Check sheet for the modelled part. Datum: model origin and axes. Units: mm. A direction names the side the tool comes from. Coordinates: 2 decimals unless noted, no trailing zeros. Loops run counter-clockwise (first coordinate to the right, second up) from the corner with the lowest first, then second, coordinate; pieces in that order, holes last.
```python
from build123d import *

# Parameters (mm, degrees)
SKETCH1_R               = 10
BOSS_EXTRUDE1_DEPTH     = 61
SKETCH3_W               = 66
SKETCH3_H               = 1.5
SKETCH4_W               = 43
SKETCH4_H               = 1.5
SKETCH5_W               = 24
SKETCH5_H               = 2.5
SKETCH6_W               = 39.5
SKETCH6_H               = 1
SKETCH7_W               = 27
SKETCH7_H               = 1.5
SKETCH8_W               = 1.1
SKETCH8_H               = 0.6
SKETCH9_W               = 1.1
SKETCH9_H               = 0.65
SKETCH10_W              = 1.1
SKETCH10_H              = 0.65
CUT_EXTRUDE1_DEPTH      = 63.617888818
CUT_EXTRUDE1_DEPTH_BACK = 63.617888818
SKETCH11_W              = 12
SKETCH11_H              = 12
CUT_EXTRUDE2_DEPTH      = 2.5


with BuildPart() as part:
    # Sketch1 → Boss-Extrude1 (new, symmetric)
    with BuildSketch(Plane.XY):
        with Locations(Location((0, 0, 0), (0, 0, 180))):
            Circle(SKETCH1_R)
    extrude(amount=BOSS_EXTRUDE1_DEPTH, both=True)

    # Sketch3 → Cut-Revolve1 (revolve, cut)
    with BuildSketch(Plane(origin=(0, 0, 0), x_dir=(0, 0, -1), z_dir=(1, 0, 0)), mode=Mode.PRIVATE) as cut_revolve1_sk:
        with Locations((28, 9.25)):
            Rectangle(SKETCH3_W, SKETCH3_H)
    revolve(cut_revolve1_sk.sketch.rotate(Axis((0, 0, 0), (0, 0, -1)), 270), axis=Axis((0, 0, 0), (0, 0, -1)), mode=Mode.SUBTRACT)

    # Sketch4 → Cut-Revolve2 (revolve, cut)
    with BuildSketch(Plane(origin=(0, 0, 0), x_dir=(0, 0, -1), z_dir=(1, 0, 0)), mode=Mode.PRIVATE) as cut_revolve2_sk:
        with Locations((-39.5, 9.25)):
            Rectangle(SKETCH4_W, SKETCH4_H)
    revolve(cut_revolve2_sk.sketch.rotate(Axis((0, 0, 0), (0, 0, 1)), 90), axis=Axis((0, 0, 0), (0, 0, 1)), mode=Mode.SUBTRACT)

    # Sketch5 → Cut-Revolve3 (revolve, cut)
    with BuildSketch(Plane(origin=(0, 0, 0), x_dir=(0, 0, -1), z_dir=(1, 0, 0)), mode=Mode.PRIVATE) as cut_revolve3_sk:
        with Locations((-49, 7.25)):
            Rectangle(SKETCH5_W, SKETCH5_H)
    revolve(cut_revolve3_sk.sketch.rotate(Axis((0, 0, 0), (0, 0, 1)), 90), axis=Axis((0, 0, 0), (0, 0, 1)), mode=Mode.SUBTRACT)

    # Sketch6 → Cut-Revolve4 (revolve, cut)
    with BuildSketch(Plane(origin=(0, 0, 0), x_dir=(0, 0, -1), z_dir=(1, 0, 0)), mode=Mode.PRIVATE) as cut_revolve4_sk:
        with Locations((41.25, 8)):
            Rectangle(SKETCH6_W, SKETCH6_H)
    revolve(cut_revolve4_sk.sketch.rotate(Axis((0, 0, 0), (0, 0, -1)), 90), axis=Axis((0, 0, 0), (0, 0, -1)), mode=Mode.SUBTRACT)

    # Sketch7 → Cut-Revolve5 (revolve, cut)
    with BuildSketch(Plane(origin=(0, 0, 0), x_dir=(0, 0, -1), z_dir=(1, 0, 0)), mode=Mode.PRIVATE) as cut_revolve5_sk:
        with Locations((47.5, 6.75)):
            Rectangle(SKETCH7_W, SKETCH7_H)
    revolve(cut_revolve5_sk.sketch.rotate(Axis((0, 0, 0), (0, 0, -1)), 90), axis=Axis((0, 0, 0), (0, 0, -1)), mode=Mode.SUBTRACT)

    # Sketch8 → Cut-Revolve6 (revolve, cut)
    with BuildSketch(Plane(origin=(0, 0, 0), x_dir=(0, 0, -1), z_dir=(1, 0, 0)), mode=Mode.PRIVATE) as cut_revolve6_sk:
        with Locations((30.95, 7.2)):
            Rectangle(SKETCH8_W, SKETCH8_H)
    revolve(cut_revolve6_sk.sketch.rotate(Axis((0, 0, 0), (0, 0, -1)), 90), axis=Axis((0, 0, 0), (0, 0, -1)), mode=Mode.SUBTRACT)

    # Sketch9 → Cut-Revolve7 (revolve, cut)
    with BuildSketch(Plane(origin=(0, 0, 0), x_dir=(0, 0, -1), z_dir=(1, 0, 0)), mode=Mode.PRIVATE) as cut_revolve7_sk:
        with Locations((5.45, 8.175)):
            Rectangle(SKETCH9_W, SKETCH9_H)
    revolve(cut_revolve7_sk.sketch.rotate(Axis((0, 0, 0), (0, 0, -1)), 90), axis=Axis((0, 0, 0), (0, 0, -1)), mode=Mode.SUBTRACT)

    # Sketch10 → Cut-Revolve8 (revolve, cut)
    with BuildSketch(Plane(origin=(0, 0, 0), x_dir=(0, 0, -1), z_dir=(1, 0, 0)), mode=Mode.PRIVATE) as cut_revolve8_sk:
        with Locations((-34.45, 8.175)):
            Rectangle(SKETCH10_W, SKETCH10_H)
    revolve(cut_revolve8_sk.sketch.rotate(Axis((0, 0, 0), (0, 0, 1)), 90), axis=Axis((0, 0, 0), (0, 0, 1)), mode=Mode.SUBTRACT)

    # Sketch11 → Cut-Extrude1 (cut, two sides: drawn at the far end of the back side and taken through both)
    with BuildSketch(Plane(origin=(0, 0, 0), x_dir=(0, 0, -1), z_dir=(1, 0, 0)).offset(-CUT_EXTRUDE1_DEPTH_BACK)):
        with Locations((55, 0)):
            Rectangle(SKETCH11_W, SKETCH11_H)
    extrude(amount=CUT_EXTRUDE1_DEPTH + CUT_EXTRUDE1_DEPTH_BACK, mode=Mode.SUBTRACT)

    # Sketch12 → Cut-Extrude2 (cut)
    with BuildSketch(Plane(origin=(0, 8.5, 0), x_dir=(1, 0, 0), z_dir=(0, 1, 0))):
        with BuildLine():
            Line((2, -31.5), (2, -20.5))
            ThreePointArc((2, -20.5), (0, -18.5), (-2, -20.5))
            Line((-2, -20.5), (-2, -31.5))
            ThreePointArc((-2, -31.5), (0, -33.5), (2, -31.5))
        make_face()
    extrude(amount=-CUT_EXTRUDE2_DEPTH, mode=Mode.SUBTRACT)


solid = part.part
```
1) Set-up check for faces 1 (the flat face through (-7, 2, -31.5)), 2 (the flat face through (-4.5, 7.4, 18)), 3 (the cylindrical face through (5.723, -1.802, -41.605)): record each of +Z, -Z, +X, -X, +Y, -Y from which the full face is reachable in a straight line by a thin tool's end or side.
Answer sheet:
face 1: none
face 2: +Z
face 3: -Z
2) Section check B-B on z = 43. Enter the section's corners in (x, y).
Answer sheet:
outline: circle Ø12 at (0, 0)
3) Section check A-A on z = -2.5. Enter the section's corners in (x, y).
Answer sheet:
outline: circle Ø17 at (0, 0)
4) Scan lines: line 1 (Z direction, x = 2.25, y = -8); line 2 (Z direction, x = 9, y = 1); line 3 (X direction, y = 0.25, z = 44). Record each from-to range of solid material in increasing order.
Answer sheet:
line 1: z = -21.5 to -6, -4.9 to 33.9, 35 to 37
line 2: z = 5 to 18
line 3: x = -5.99 to 5.99
5) Depth check by flat-ended pin: pin 1 (8 mm diameter, centred on x = 0, z = 30, fed in from -Y); pin 2 (8 mm diameter, centred on y = 6.5, z = 6.5, fed in from +X); pin 3 (1 mm diameter, centred on x = 7, y = -4.5, fed in from -Z). Enter the tip coordinate at first touch or a pass-through.
Answer sheet:
pin 1: stops at y = -8.5
pin 2: stops at x = 9.68
pin 3: stops at z = -21.5
6) Mould release check, pull along X, two halves, no side actions. Record for faces 4 (the flat face through (-2, 7, 26)), 5 (the flat face through (8, 2, 35)), 6 (the cylindrical face through (10, 0, 12)): +X half, -X half, draft (parallel to the pull), parting line (faces both ways), or undercut.
Answer sheet:
face 4: undercut
face 5: draft
face 6: parting line
